Input: part model. Units: mm. Frame: model coordinates. A direction names the side the tool comes from. Coordinates: 2 decimals unless noted, no trailing zeros. Loops run counter-clockwise (first coordinate to the right, second up) from the corner with the lowest first, then second, coordinate; pieces in that order, holes last. Notation, with made-up numbers: (32, 9.5) -> (46, 9.5) arc R22 cw to (46, 24.5) -> close; hole circle Ø3 at (21.25, 73). An arc over 180 degrees is marked (long way). Answer as a JSON object with one key per item and string values.
from build123d import *

# Parameters (mm, degrees)
SKETCH_1_R          = 7.25
EXTRUDE_1_DEPTH     = 1.5
EXTRUDE_2_DEPTH     = 1.5
FILLET_1_R          = 0.5
CUT_EXTRUDE_1_REACH = 21.305
SKETCH_3_R          = 2
EXTRUDE_START       = 1.5
SKETCH_4_R          = 2.75
SKETCH_4_R_2        = 2
EXTRUDE_3_DEPTH     = 1.5
CUT_EXTRUDE_2_REACH = 22.241
SKETCH_6_R          = 1
EXTRUDE_4_DEPTH     = 2
SKETCH_7_R          = 1.25
SKETCH_8_R          = 0.75
EXTRUDE_START_2     = 2
SKETCH_9_R          = 1
SKETCH_9_W          = 1
SKETCH_9_H          = 5
EXTRUDE_5_DEPTH     = 2
SKETCH_10_R         = 3
EXTRUDE_6_DEPTH     = 1
SKETCH_11_R         = 2
EXTRUDE_7_DEPTH     = 9
SKETCH_12_R         = 2.1
SKETCH_13_R         = 1.8
SKETCH_14_W         = 8
SKETCH_14_H         = 0.8
CUT_EXTRUDE_3_DEPTH = 6


# Read off the part's stored shape, not the designer's step: 镜向1
with BuildPart() as part:
    # 草图1 → 凸台-拉伸1 (new body)
    with BuildSketch(Plane(origin=(0, 0, 0), x_dir=(1, 0, 0), z_dir=(0, 1, 0))):
        with Locations(Location((0, 0, 0), (0, 0, 270))):
            Circle(SKETCH_1_R)
    extrude(amount=EXTRUDE_1_DEPTH)

    # 草图2 → 凸台-拉伸2 (add)
    with BuildSketch(Plane(origin=(3.5, 0, 0), x_dir=(0, 0, -1), z_dir=(1, 0, 0))):
        with BuildLine():
            Line((0, 0), (-3.5, 0))
            Line((-3.5, 0), (-3.5, 6.5))
            ThreePointArc((-3.5, 6.5), (0, 10), (3.5, 6.5))
            Line((3.5, 6.5), (3.5, 2.156854249))
            Line((3.5, 2.156854249), (9.121320344, 7.778174593))
            ThreePointArc((9.121320344, 7.778174593), (11.949747468, 7.778174593), (11.949747468, 4.949747468))
            Line((11.949747468, 4.949747468), (7, 0))
            Line((7, 0), (0, 0))
        make_face()
    extrude(amount=-EXTRUDE_2_DEPTH)

    # 圆角1
    fillet_1_edges = [part.edges().sort_by_distance(p)[0] for p in [
        (2.75, 2.156854249, -3.5),
    ]]
    fillet(fillet_1_edges, radius=FILLET_1_R)

    # 草图3 → 切除-拉伸1 (cut, up to next)
    with BuildSketch(Plane(origin=(3.5, 0, 0), x_dir=(0, 0, -1), z_dir=(1, 0, 0)), mode=Mode.PRIVATE) as cut_extrude_1_sk1:
        with Locations((0, 6.5)):
            Circle(SKETCH_3_R)
    cut_extrude_1_tool1 = extrude(cut_extrude_1_sk1.sketch, amount=-CUT_EXTRUDE_1_REACH, mode=Mode.PRIVATE) & part.part
    add(cut_extrude_1_tool1.solids().sort_by_distance((3.5, 6.5, 0))[0], mode=Mode.SUBTRACT)

    # 草图4 → 凸台-拉伸3 (add)
    with BuildSketch(Plane(origin=(3.5, 0, 0), x_dir=(0, 0, -1), z_dir=(1, 0, 0)).offset(EXTRUDE_START)):
        with Locations((0, 6.5)):
            Circle(SKETCH_4_R)
        with Locations((0, 6.5)):
            Circle(SKETCH_4_R_2, mode=Mode.SUBTRACT)
    extrude(amount=-EXTRUDE_3_DEPTH)

    # 草图5 → 切除-拉伸2 (cut, up to next)
    with BuildSketch(Plane.XY.offset(3.5), mode=Mode.PRIVATE) as cut_extrude_2_sk1:
        Polygon((5, 9.25), (4, 9.25), (5, 3.75), align=None)
    cut_extrude_2_tool1 = extrude(cut_extrude_2_sk1.sketch, amount=-CUT_EXTRUDE_2_REACH, mode=Mode.PRIVATE) & part.part
    add(cut_extrude_2_tool1.solids().sort_by_distance((4.666667, 7.416667, 3.5))[0], mode=Mode.SUBTRACT)

    # 草图6 → 凸台-拉伸4 (add)
    with BuildSketch(Plane(origin=(3.5, 0, 0), x_dir=(0, 0, -1), z_dir=(1, 0, 0))):
        with Locations((10.535533906, 6.363961031)):
            Circle(SKETCH_6_R)
    extrude(amount=EXTRUDE_4_DEPTH)

    # 草图7 → 放样1 section 0
    with BuildSketch(Plane(origin=(5.5, 0, 0), x_dir=(0, 0, -1), z_dir=(1, 0, 0))):
        with Locations((10.535533906, 6.363961031)):
            Circle(SKETCH_7_R)
    # 草图8 → 放样1 section 1
    with BuildSketch(Plane(origin=(7, 0, 0), x_dir=(0, 0, -1), z_dir=(1, 0, 0))):
        with Locations((10.535533906, 6.363961031)):
            Circle(SKETCH_8_R)
    loft()

    # 草图9 → 凸台-拉伸5 (add)
    with BuildSketch(Plane.ZY.offset(-2).offset(EXTRUDE_START_2)):
        with Locations(Location((-10.535533906, 6.363961031, 0), (0, 0, 180))):
            Circle(SKETCH_9_R)
        with Locations((3, 4)):
            Rectangle(SKETCH_9_W, SKETCH_9_H)
        with Locations((-3, 4)):
            Rectangle(SKETCH_9_W, SKETCH_9_H)
    extrude(amount=-EXTRUDE_5_DEPTH)

    # 镜向1: part across plane


with BuildPart() as part_1:
    add(part.part)
    add(part.part.mirror(Plane(origin=(0, 0, 0), x_dir=(0, 0, 1), z_dir=(1, 0, 0))))

    # 草图10 → 凸台-拉伸6 (add)
    with BuildSketch(Plane.XZ):
        with Locations(Location((0, 0, 0), (0, 0, 90))):
            Circle(SKETCH_10_R)
    extrude(amount=EXTRUDE_6_DEPTH)

    # 草图11 → 凸台-拉伸7 (add)
    with BuildSketch(Plane.XZ.offset(1)):
        with Locations(Location((0, 0, 0), (0, 0, 270))):
            Circle(SKETCH_11_R)
    extrude(amount=EXTRUDE_7_DEPTH)

    # 草图12 → 放样2 section 0
    with BuildSketch(Plane.XZ.offset(10)):
        Circle(SKETCH_12_R)
    # 草图13 → 放样2 section 1
    with BuildSketch(Plane(origin=(0, -11, 0), x_dir=(-1, 0, 0), z_dir=(0, -1, 0))):
        Circle(SKETCH_13_R)
    loft()

    # 草图14 → 切除-拉伸3 (cut)
    with BuildSketch(Plane.XZ.offset(11)):
        Rectangle(SKETCH_14_W, SKETCH_14_H)
    extrude(amount=-CUT_EXTRUDE_3_DEPTH, mode=Mode.SUBTRACT)


solid = part_1.part
1. Access query for faces 1 (the face through (-1.774, -5.437, -0.923)), 2 (the face through (0, 1.5, 5)), 3 (the face through (0, 4, 3.5)), 4 (the face through (4.094, 3.815, 0.596)). Directions: +Z, -Z, +X, -X, +Y, -Y. A direction counts if a zero-diameter tool reaches every point of the face in a straight line with its end or side. Return the directions, or none.
Reply:
{"face 1": "none", "face 2": "+Z", "face 3": "+Z, +X, -X, +Y", "face 4": "+X"}
2. Section query A-A (y = 1). Return loops of the section in (x, z).
Reply:
{"outline": "(-3.5, -8) -> (-2, -8) -> (-2, -6.97) arc R7.25 ccw to (2, -6.97) -> (2, -8) -> (3.5, -8) -> (3.5, -6.35) arc R7.25 ccw (long way) to (-3.5, -6.35) -> close"}
3. Section query B-B (z = 0). Count the separate pieces of the cut face and the enclosed holes in it, plus the area to 4 significant figures.
Reply:
{"separate pieces": "3", "enclosed holes": "0", "area": "60.25 mm2"}
4. Pin query (flat end, axial travel): P1, Ø4.5, axis at y = 6.5, z = 0, coming from the +X side; P2, Ø0.5, axis at x = 0.5, z = 1.5, coming from the +Y side; P3, Ø6.5, axis at y = 5.5, z = -10, coming from the +X side. Return the tip coordinate at first contact, or that it passes through.
Reply:
{"P1": "stops at x = 4.91", "P2": "stops at y = 1.5", "P3": "stops at x = 7"}
5. Mould query, pull axis Z, two halves, no side actions, for faces 5 (the face through (-3, 3, -10)), 6 (the face through (-2.76, 5.361, -6.704)), 7 (the face through (0, 1.5, 0)), 8 (the face through (6.594, 6.025, -11.353)). Classes: pulls with the +Z half, pulls with the -Z half, needs draft (parallel to the pull), parting line crosses it, or undercut.
Reply:
{"face 5": "pulls with the -Z half", "face 6": "undercut", "face 7": "undercut", "face 8": "parting line crosses it"}
6. Line query: line 1 along Y through (x, z) = (-3.7, 0); line 2 along Z through (x, y) = (3, 6.5); line 3 along Y through (x, z) = (-2.95, 0). Output: solid intervals per line, ascending.
Reply:
{"line 1": "y = 0 to 1.5, 3.75 to 4.5, 8.5 to 9.25", "line 2": "z = -12.53 to -7.84, -3.5 to -2, 2 to 3.5", "line 3": "y = -1 to 4.5, 8.5 to 10"}
7. Section query D-D (y = -9.25). Return loops of the section in (x, z), plus the area to 3 significant figures.
Reply:
{"outline": "(-1.96, -0.4) arc R2 ccw to (1.96, -0.4) -> close; (-1.96, 0.4) -> (1.96, 0.4) arc R2 ccw to start", "area": "9.39 mm2"}
